```python
from build123d import *

# Parameters (mm, degrees)
CROQUIS1_W             = 112
CROQUIS1_H             = 132
BRIDA_BASE1_DEPTH      = 0.5
CORTAR_EXTRUIR4_DEPTH  = 10
CROQUIS7_R             = 1.5
CORTAR_EXTRUIR5_DEPTH  = 10
CORTAR_EXTRUIR6_DEPTH  = 10
CROQUIS9_R             = 1.5
CORTAR_EXTRUIR7_DEPTH  = 12
CROQUIS10_R            = 1.5
CORTAR_EXTRUIR8_DEPTH  = 10
CROQUIS11_R            = 1.5
CORTAR_EXTRUIR9_DEPTH  = 10
CROQUIS12_W            = 6
CROQUIS12_H            = 6
CORTAR_EXTRUIR10_DEPTH = 10
CROQUIS13_R            = 5
CORTAR_EXTRUIR11_DEPTH = 10


# Sheet-metal steps are written as plain solids
with BuildPart() as part:
    # Croquis1 → Brida base1 (new body)
    with BuildSketch(Plane(origin=(0, 0, 0), x_dir=(1, 0, 0), z_dir=(0, 1, 0))):
        Rectangle(CROQUIS1_W, CROQUIS1_H)
    extrude(amount=-BRIDA_BASE1_DEPTH)

    # Croquis5 → Cortar-Extruir4 (cut)
    with BuildSketch(Plane(origin=(0, 0, 0), x_dir=(1, 0, 0), z_dir=(0, 1, 0))):
        Polygon((-15.25, 61), (-15.25, 66), (-56, 66), (-56, 54), (-25.5, 54), (-25.5, 61), align=None)
        Polygon((56, 66), (15.25, 66), (15.25, 61), (25.5, 61), (25.5, 54), (56, 54), align=None)
    extrude(amount=-CORTAR_EXTRUIR4_DEPTH, mode=Mode.SUBTRACT)

    # Croquis7 → Cortar-Extruir5 (cut)
    with BuildSketch(Plane(origin=(0, 0, 0), x_dir=(1, 0, 0), z_dir=(0, 1, 0))):
        with Locations(Location((-40.75, -4.5, 0), (0, 0, 270))):
            Circle(CROQUIS7_R)
        with Locations(Location((40.75, -4.5, 0), (0, 0, 90))):
            Circle(CROQUIS7_R)
        with Locations(Location((0, 7.5, 0), (0, 0, 270))):
            Circle(CROQUIS7_R)
    extrude(amount=-CORTAR_EXTRUIR5_DEPTH, mode=Mode.SUBTRACT)

    # Croquis8 → Cortar-Extruir6 (cut)
    with BuildSketch(Plane(origin=(0, 0, 0), x_dir=(1, 0, 0), z_dir=(0, 1, 0))):
        Polygon((-56, -17.588089006), (-56, -41), (-21.238275218, -53.652233112), (-19.528174501, -48.953770009), (-28.925100709, -45.533568575), (-23.110758272, -29.558794022), align=None)
    extrude(amount=-CORTAR_EXTRUIR6_DEPTH, mode=Mode.SUBTRACT)

    # Croquis9 → Cortar-Extruir7 (cut)
    with BuildSketch(Plane(origin=(0, 0, 0), x_dir=(1, 0, 0), z_dir=(0, 1, 0))):
        with Locations(Location((-13, 60, 0), (0, 0, 270))):
            Circle(CROQUIS9_R)
        with Locations(Location((13, 60, 0), (0, 0, 90))):
            Circle(CROQUIS9_R)
        with Locations(Location((-53.75, 48, 0), (0, 0, 270))):
            Circle(CROQUIS9_R)
        with Locations(Location((-27.75, 48, 0), (0, 0, 90))):
            Circle(CROQUIS9_R)
        with Locations(Location((27.75, 48, 0), (0, 0, 270))):
            Circle(CROQUIS9_R)
        with Locations(Location((53.75, 48, 0), (0, 0, 90))):
            Circle(CROQUIS9_R)
    extrude(amount=-CORTAR_EXTRUIR7_DEPTH, mode=Mode.SUBTRACT)

    # Croquis10 → Cortar-Extruir8 (cut)
    with BuildSketch(Plane(origin=(0, 0, 0), x_dir=(1, 0, 0), z_dir=(0, 1, 0))):
        with Locations(Location((-37.346445111, -18.977085256, 0), (0, 0, 270))):
            Circle(CROQUIS10_R)
        with Locations(Location((-26.070133662, -23.081326976, 0), (0, 0, 90))):
            Circle(CROQUIS10_R)
        with Locations(Location((-37.065850057, -53.291809483, 0), (0, 0, 270))):
            Circle(CROQUIS10_R)
        with Locations(Location((-48.342161507, -49.187567763, 0), (0, 0, 90))):
            Circle(CROQUIS10_R)
    extrude(amount=-CORTAR_EXTRUIR8_DEPTH, mode=Mode.SUBTRACT)

    # Croquis11 → Cortar-Extruir9 (cut)
    with BuildSketch(Plane(origin=(0, 0, 0), x_dir=(1, 0, 0), z_dir=(0, 1, 0))):
        with Locations(Location((-10, -61, 0), (0, 0, 270))):
            Circle(CROQUIS11_R)
        with Locations(Location((-30, -61, 0), (0, 0, 270))):
            Circle(CROQUIS11_R)
        with Locations(Location((30, -61, 0), (0, 0, 90))):
            Circle(CROQUIS11_R)
        with Locations(Location((10, -61, 0), (0, 0, 90))):
            Circle(CROQUIS11_R)
        with Locations(Location((-51, -61, 0), (0, 0, 270))):
            Circle(CROQUIS11_R)
        with Locations(Location((51, -61, 0), (0, 0, 90))):
            Circle(CROQUIS11_R)
    extrude(amount=-CORTAR_EXTRUIR9_DEPTH, mode=Mode.SUBTRACT)

    # Croquis12 → Cortar-Extruir10 (cut)
    with BuildSketch(Plane(origin=(0, 0, 0), x_dir=(1, 0, 0), z_dir=(0, 1, 0))):
        with Locations((0, -63)):
            Rectangle(CROQUIS12_W, CROQUIS12_H)
    extrude(amount=-CORTAR_EXTRUIR10_DEPTH, mode=Mode.SUBTRACT)

    # Croquis13 → Cortar-Extruir11 (cut)
    with BuildSketch(Plane(origin=(0, 0, 0), x_dir=(1, 0, 0), z_dir=(0, 1, 0))):
        with Locations(Location((-20.375, -2.011448093, 0), (0, 0, 270))):
            Circle(CROQUIS13_R)
        with Locations(Location((20.375, -0.670482698, 0), (0, 0, 270))):
            Circle(CROQUIS13_R)
    extrude(amount=-CORTAR_EXTRUIR11_DEPTH, mode=Mode.SUBTRACT)


solid = part.part
```
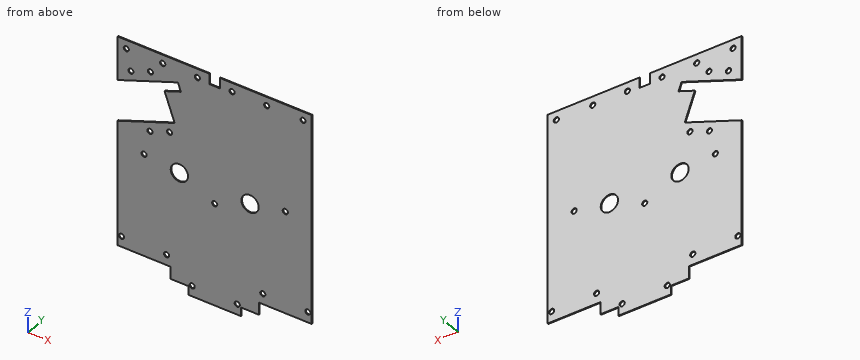
Geometry check sheet. Reference: the model listing, model coordinates, mm. Coordinates: 2 decimals unless noted, no trailing zeros. Write each loop counter-clockwise with the first axis right and the second up, starting at its lowest first coordinate (ties: lowest second). Pieces come first, ordered by that corner, then holes. Notation, with made-up numbers: (28.5, 63) -> (59.5, 63) arc R7 cw to (59.5, 74) -> close; hole circle Ø7 at (2, 70). An arc over 180 degrees is marked (long way). Use CSV: the item, a comma, the result in double quotes. Start each with the question number.
Item 1: Cross-section at C-C, the plane y = -0.35. State how many separate pieces and enclosed holes the cut face has, plus the area to 3 significant figures.
Item 2: Cross-section at A-A, the plane x = 0. Record the cut outline in (y, z), plus the area to 3 significant figures.
Item 3: Thickness scan on line 1 (Z direction, x = -37, y = -0.2); line 2 (Z direction, x = 41, y = -0.3); line 3 (X direction, y = -0.4, z = -47.5). Record the ranges inside material, lowest first.
Item 4: Cross-section at D-D, the plane z = 28. Record the cut outline in (x, y), plus the area to 3 significant figures.
Item 5: Cross-section at B-B, the plane x = 13. Record the cut outline in (y, z), plus the area to 3 significant figures.
Answers:
1,separate pieces,"1"
1,enclosed holes,"21"
1,area,"12,900 mm^2"
2,outline,"(-0.5, -66) -> (0, -66) -> (0, -9) -> (-0.5, -9) -> close; (-0.5, -6) -> (0, -6) -> (0, 60) -> (-0.5, 60) -> close"
2,area,"61.5 mm^2"
3,line 1,"-54 to 17.52, 20.44 to 24.5, 47.92 to 51.79, 54.79 to 66"
3,line 2,"-54 to 3.02, 5.98 to 66"
3,line 3,"-56 to -55.16, -52.34 to -29.16, -26.34 to 26.34, 29.16 to 52.34, 55.16 to 56"
4,outline,"(-27.39, -0.5) -> (56, -0.5) -> (56, 0) -> (-27.39, 0) -> close"
4,area,"41.7 mm^2"
5,outline,"(-0.5, -66) -> (0, -66) -> (0, -61.5) -> (-0.5, -61.5) -> close; (-0.5, -58.5) -> (0, -58.5) -> (0, 66) -> (-0.5, 66) -> close"
5,area,"64.5 mm^2"
